Answer from the drawing. Dimensions are ordinates in mm from the lowest x, y and z of the part. Give positions to 0.01 mm unless a question says otherwise; leave off trailing zeros. Order: outer loops, then holes, each group sorted by start corner. A loop starts at its lowest first (then second) coordinate and runs counter-clockwise, first axis right, second up. Notation, with made-up numbers: (57.25, 87.25) - (63.25, 87.25) arc R17 cw to (63.25, 98.25) - close; hole circle Ø7 at (-8.75, 41.5). An arc over 180 degrees is marked (long way). Write each question's results on one line, items separated by ' | '.
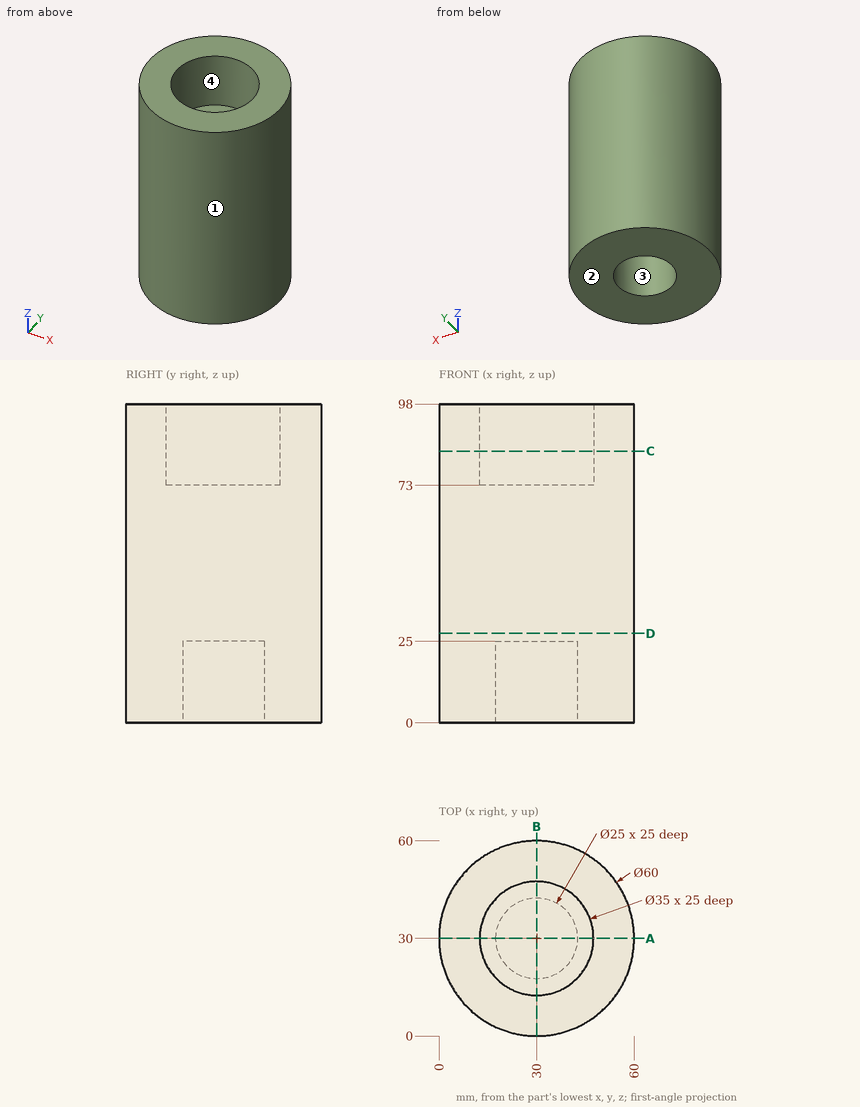
(1) Each of these flat-tipped pins is pushed along its axis until it touches: pin 1 (2 mm diameter, centred on x = 46.5, z = 55, fed in from -Y); pin 2 (4 mm diameter, centred on x = 22, z = 13.5, fed in from +Y); pin 3 (6 mm diameter, centred on x = 52.5, z = 80, fed in from -Y); pin 4 (10 mm diameter, centred on x = 35, y = 40, fed in from -Z). Where does it stop, or does it pass through?
Conclusion:
pin 1: y = 4.31 | pin 2: y = 59.39 | pin 3: y = 7.2 | pin 4: z = 0
(2) Consider probe 1 along X at (y, z) = (30.5, 23.5); probe 2 along Y at (x, z) = (30, 13.5); probe 3 along Y at (x, z) = (30, 81.5). Determine where each line is inside the solid, lowest interval first. Write a range as [from, to].
Conclusion:
probe 1: [0, 17.51], [42.49, 60] | probe 2: [0, 17.5], [42.5, 60] | probe 3: [0, 12.5], [47.5, 60]
(3) Section D-D (z = 27.5) is taken. Give the vertices of the cut face in (x, y), plus the area to 3 significant figures.
Conclusion:
outline: circle Ø60 at (30, 30) | area: 2,830 mm^2
(4) Section A-A (y = 30) is taken. Give the vertices of the cut face in (x, z).
Conclusion:
outline: (0, 0) - (17.5, 0) - (17.5, 25) - (42.5, 25) - (42.5, 0) - (60, 0) - (60, 98) - (47.5, 98) - (47.5, 73) - (12.5, 73) - (12.5, 98) - (0, 98) - close
(5) Section C-C (z = 83.5) is taken. Give the vertices of the cut face in (x, y), plus the area to 3 significant figures.
Conclusion:
outline: circle Ø60 at (30, 30); hole circle Ø35 at (30, 30) | area: 1,870 mm^2
(6) The mould has two halves that part along X. Classify the marked faces 1, 2, 3 and 4: pulls with the +X half, pulls with the -X half, needs draft (parallel to the pull), parting line crosses it, or undercut.
Conclusion:
face 1: parting line crosses it | face 2: needs draft | face 3: undercut | face 4: undercut
